Build history of the part. All positions in model axes, mm. Face numbers are marked on the shaded views. A direction names the side the tool comes from. Coordinates: 2 decimals unless noted, no trailing zeros. Order: outer loops, then holes, each group sorted by start corner. A loop starts at its lowest first (then second) coordinate and runs counter-clockwise, first axis right, second up. Notation, with made-up numbers: M 68.25,68.25 L 81.25,68.25 A19 cw 81.25,86.25 Z; hole C 66,44.5 d2. An arc over 180 degrees is marked long. Use a Markdown table: item, result. Add a question column.
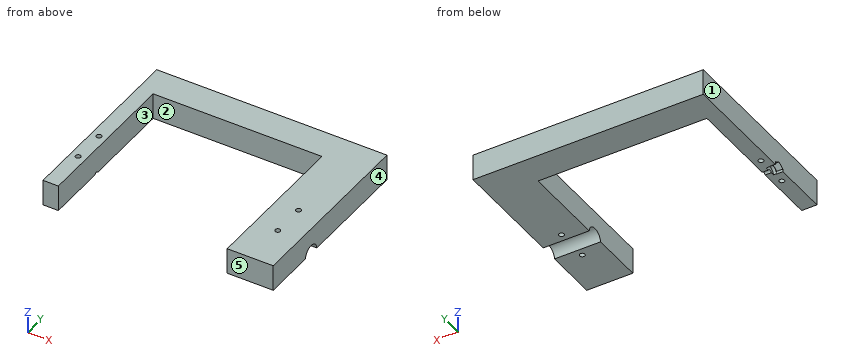
from build123d import *

# Parameters (mm, degrees)
F0_W      = 150
F0_H      = 120
F1_DEPTH  = 30
F3_W      = 110
F3_H      = 100
F4_DEPTH  = 30
F5_DEPTH  = 4
F6_R      = 3.8
F7_DEPTH  = 2
F8_R      = 1.55
F9_DEPTH  = 7
F10_R     = 6
F12_DEPTH = 30
F11_R     = 0.5
F13_DEPTH = 1
F14_W     = 150
F14_H     = 120
F15_DEPTH = 13
F16_R     = 1.65
F17_DEPTH = 30


with BuildPart() as f1:
    # F0 (on Top) → F1 (new body)
    with BuildSketch(Plane.XY):
        Rectangle(F0_W, F0_H)
    extrude(amount=F1_DEPTH)

    # F3 (on Top) → F4 (cut, through all)
    with BuildSketch(Plane.XY):
        with Locations((-10, -10)):
            Rectangle(F3_W, F3_H)
    extrude(amount=F4_DEPTH, mode=Mode.SUBTRACT)

    # F2 (on face) → F5 (cut)
    with BuildSketch(Plane(origin=(-75, 0, 0), x_dir=(0, -1, 0), z_dir=(-1, 0, 0))):
        Polygon((20, 17.12), (15.998963, 14.81), (15.998963, 10.19), (20, 7.88), (24.001037, 10.19), (24.001037, 14.81), align=None)
    extrude(amount=-F5_DEPTH, mode=Mode.SUBTRACT)

    # F6 (on face) → F7 (cut)
    with BuildSketch(Plane(origin=(-71, 0, 0), x_dir=(0, -1, 0), z_dir=(-1, 0, 0))):
        with Locations((20, 12.5)):
            Circle(F6_R)
    extrude(amount=-F7_DEPTH, mode=Mode.SUBTRACT)

    # F8 (on face) → F9 (cut)
    with BuildSketch(Plane(origin=(-69, 0, 0), x_dir=(0, -1, 0), z_dir=(-1, 0, 0))):
        with Locations((20, 12.5)):
            Circle(F8_R)
    extrude(amount=-F9_DEPTH, mode=Mode.SUBTRACT)

    # F10 (on face) → F12 (cut, through all)
    with BuildSketch(Plane.YZ.offset(75)):
        with Locations((-20, 12.5)):
            Circle(F10_R)
    extrude(amount=-F12_DEPTH, mode=Mode.SUBTRACT)

    # F11 (on face) → F13 (cut)
    with BuildSketch(Plane(origin=(0, 60, 0), x_dir=(-1, 0, 0), z_dir=(0, 1, 0))):
        with Locations((20, 6)):
            Circle(F11_R)
        with Locations((-5, 6)):
            Circle(F11_R)
    extrude(amount=-F13_DEPTH, mode=Mode.SUBTRACT)

    # F14 (on Top) → F15 (cut)
    with BuildSketch(Plane.XY):
        Rectangle(F14_W, F14_H)
    extrude(amount=F15_DEPTH, mode=Mode.SUBTRACT)

    # F16 (on Top) → F17 (cut, through all)
    with BuildSketch(Plane.XY):
        with Locations((-70, -9)):
            Circle(F16_R)
        with Locations((-70, -31)):
            Circle(F16_R)
        with Locations((60, -9)):
            Circle(F16_R)
        with Locations((60, -31)):
            Circle(F16_R)
    extrude(amount=F17_DEPTH, mode=Mode.SUBTRACT)


solid = f1.part
(1) Which spindle directions (+Z, -Z, +X, -X, +Y, -Y) get a long thin tool onto all of the face, cutting with end or side? Do the marked faces 1 and 2. Say none if no direction does.
(2) Slice it at B-B on x = 60. Give the cut face in (y, z).
(3) Drill centre lines: line 1 along X through (y, z) = (-31, 24.25); line 2 along Y through (x, z) = (-70, 20.25); line 3 along X through (y, z) = (-38, 26.5). Where is each one in solid material? Low to high. Write a range as from..to.
(4) Slice it at A-A on y = -51.5. Give the cut face in (x, z), and give its area (3 significant figures).
(5) Mould opens along X. For the marked faces 3, 4 and 5 say: released by +X, released by -X, zero draft, split by the parting line, or undercut.
(6) Slice it at C-C on y = -9. Give the cut face in (x, z).
(7) Slice it at D-D on z = 20.5. Give the cut face in (x, y).
(8) Drop flat-ended pins along their axis: P1, Ø1.5, axis at x = -33, z = 19.5, coming from the -Y side; P2, Ø4.5, axis at x = -70, y = -31, coming from the +Z side; P3, Ø2, axis at x = 60, y = -9, coming from the -Z side; P4, Ø1, axis at y = -20, z = 14.5, coming from the -X side. Give the stop position or say it passes through.
Solutions:
| question | item | result |
|---|---|---|
| 1 | face 1 | +Z, -Z, -X, +Y, -Y |
| 1 | face 2 | +Z, -Z, -Y |
| 2 | outline | M -60,13 L -32.65,13 L -32.65,30 L -60,30 Z; M -29.35,13 L -25.98,13 A6 cw -14.02,13 L -10.65,13 L -10.65,30 L -29.35,30 Z; M -7.35,13 L 60,13 L 60,30 L -7.35,30 Z |
| 3 | line 1 | -75..-71.65, -68.35..-65, 45..58.35, 61.65..75 |
| 3 | line 2 | -60..-32.65, -29.35..-10.65, -7.35..60 |
| 3 | line 3 | -75..-65, 45..75 |
| 4 | outline | M -75,13 L -65,13 L -65,30 L -75,30 Z; M 45,13 L 75,13 L 75,30 L 45,30 Z |
| 4 | area | 680 mm² |
| 5 | face 3 | undercut |
| 5 | face 4 | released by +X |
| 5 | face 5 | zero draft |
| 6 | outline | M -75,13 L -71.65,13 L -71.65,30 L -75,30 Z; M -68.35,13 L -65,13 L -65,30 L -68.35,30 Z; M 45,13 L 58.35,13 L 58.35,30 L 45,30 Z; M 61.65,13 L 75,13 L 75,30 L 61.65,30 Z |
| 7 | outline | M -75,-60 L -65,-60 L -65,40 L 45,40 L 45,-60 L 75,-60 L 75,60 L -75,60 Z; hole C -70,-31 d3.3; hole C -70,-9 d3.3; hole C 60,-31 d3.3; hole C 60,-9 d3.3 |
| 8 | P1 | y = 40 |
| 8 | P2 | z = 30 |
| 8 | P3 | through |
| 8 | P4 | x = -69 |
